CAD build for the part. Positions are in the model's coordinates, mm. Face numbers are marked on the shaded views. A direction names the side the tool comes from. Coordinates: 2 decimals unless noted, no trailing zeros. Loops run counter-clockwise (first coordinate to the right, second up) from the corner with the lowest first, then second, coordinate; pieces in that order, holes last. Notation, with made-up numbers: (55.5, 13.5) -> (92.5, 13.5) arc R36 ccw to (92.5, 49.5) -> close; hole circle Ø7 at (-11.5, 29.25). An arc over 180 degrees is marked (long way). Return JSON: item names as keys, results as strings. Group by question number.
(1) Probe L1, parallel to Z at x = -4.5, y = -6; L2, parallel to Y at x = -8.5, z = 17.1; L3, parallel to X at y = 2, z = 4. List the from-to ranges inside material, lowest first.
(2) Flat gauge pins, fed straight in: pin 1 Ø2 at (y, z) = (15.5, 18) entering from +X; pin 2 Ø4 at (x, z) = (0, 10) entering from +Y; pin 3 Ø1.5 at (y, z) = (-8, 8.5) entering from +X. Where does each tip first touch, or does it go through?
(3) Saw through at B-B on z = 16.5. Write the cut outline in (x, y), then the cut area to 3 significant figures.
(4) Saw through at D-D on x = 0. Write the cut outline in (y, z), then the cut area to 3 significant figures.
(5) Mould opens along Y. For the marked faces 6, 7 and 8 say: pulls with the +Y half, pulls with the -Y half, needs draft (parallel to the pull), parting line crosses it, or undercut.
(6) Saw through at C-C on y = -3. Write the cut outline in (x, z).
(7) Saw through at A-A on x = -8.5. Write the cut outline in (y, z).
(8) Tool access for the marked faces 1, 2, 3, 4 and 5: list every direction of +Z, -Z, +X, -X, +Y, -Y with a clear straight run to the whole face (end or side of a thin tool).
```python
from build123d import *

# Parameters (mm, degrees)
SKETCH_W     = 17
SKETCH_H     = 14
SKETCH_R     = 2.5
PAD_DEPTH    = 3
SKETCH001_W  = 3
SKETCH001_H  = 14
PAD001_DEPTH = 16
SKETCH002_W  = 14
SKETCH002_H  = 3
PAD002_DEPTH = 13
SKETCH003_W  = 34
SKETCH003_H  = 3
PAD003_DEPTH = 9
SKETCH004_W  = 14
SKETCH004_H  = 3
PAD004_DEPTH = 8
SKETCH006_R  = 2
POCKET_DEPTH = 19.001
PAD005_DEPTH = 3
SKETCH008_W  = 23
SKETCH008_H  = 19
PAD006_DEPTH = 3
SKETCH009_W  = 3
SKETCH009_H  = 19
PAD007_DEPTH = 4
CHAMFER_SIZE = 2.9
FILLET_R     = 2
FILLET001_R  = 2
FILLET002_R  = 0.5


with BuildPart() as part:
    # Sketch → Pad (new body)
    with BuildSketch(Plane.XY):
        with Locations((3.5, 0)):
            Rectangle(SKETCH_W, SKETCH_H)
        Circle(SKETCH_R, mode=Mode.SUBTRACT)
    extrude(amount=PAD_DEPTH)

    # Sketch001 (on Face7 of Pad) → Pad001 (join)
    with BuildSketch(Plane.XY.offset(3)):
        with Locations((10.5, 0)):
            Rectangle(SKETCH001_W, SKETCH001_H)
    extrude(amount=PAD001_DEPTH)

    # Sketch002 (on Face10 of Pad001) → Pad002 (join)
    with BuildSketch(Plane(origin=(9, 0, 0), x_dir=(0, -1, 0), z_dir=(-1, 0, 0))):
        with Locations((0, 17.5)):
            Rectangle(SKETCH002_W, SKETCH002_H)
    extrude(amount=PAD002_DEPTH)

    # Sketch003 (on Face16 of Pad002) → Pad003 (join)
    with BuildSketch(Plane(origin=(-4, 0, 0), x_dir=(0, -1, 0), z_dir=(-1, 0, 0))):
        with Locations((-10, 17.5)):
            Rectangle(SKETCH003_W, SKETCH003_H)
    extrude(amount=PAD003_DEPTH)

    # Sketch004 (on Face2 of Pad003) → Pad004 (join)
    with BuildSketch(Plane(origin=(-5, 0, 0), x_dir=(0, -1, 0), z_dir=(-1, 0, 0))):
        with Locations((0, 1.5)):
            Rectangle(SKETCH004_W, SKETCH004_H)
    extrude(amount=PAD004_DEPTH)

    # Sketch006 → Pocket (cut, through all)
    with BuildSketch(Plane.XY.offset(19)):
        with Locations((-8.5, 22)):
            Circle(SKETCH006_R)
        with Locations((-8.5, 12)):
            Circle(SKETCH006_R)
    extrude(amount=-POCKET_DEPTH, mode=Mode.SUBTRACT)

    # Sketch007 (on Face26 of Pocket) → Pad005 (join)
    with BuildSketch(Plane(origin=(-13, 0, 0), x_dir=(0, -1, 0), z_dir=(-1, 0, 0))):
        Polygon((-27, 19), (7, 19), (7, 0), (-7, 0), (-27, 16), align=None)
    extrude(amount=PAD005_DEPTH)

    # Sketch008 (on Face10 of Pad005) → Pad006 (join)
    with BuildSketch(Plane.XZ.offset(7)):
        with Locations((-4.5, 9.5)):
            Rectangle(SKETCH008_W, SKETCH008_H)
    extrude(amount=PAD006_DEPTH)

    # Sketch009 (on Face15 of Pad006) → Pad007 (join)
    with BuildSketch(Plane(origin=(9, 0, 0), x_dir=(0, -1, 0), z_dir=(-1, 0, 0))):
        with Locations((5.5, 9.5)):
            Rectangle(SKETCH009_W, SKETCH009_H)
    extrude(amount=PAD007_DEPTH)

    # Chamfer
    chamfer_edges = [part.edges().sort_by_distance(p)[0] for p in [
        (5, -4, 9.5),
    ]]
    chamfer(chamfer_edges, length=CHAMFER_SIZE)

    # Fillet
    fillet_edges = [part.edges().sort_by_distance(p)[0] for p in [
        (-4, 27, 17.5),
    ]]
    fillet(fillet_edges, radius=FILLET_R)

    # Fillet001
    fillet001_edges = [part.edges().sort_by_distance(p)[0] for p in [
        (-16, 27, 17.5),
    ]]
    fillet(fillet001_edges, radius=FILLET001_R)

    # Fillet002
    fillet002_edges = [part.edges().sort_by_distance(p)[0] for p in [
        (-16, 9, 19),
    ]]
    fillet(fillet002_edges, radius=FILLET002_R)


solid = part.part
```
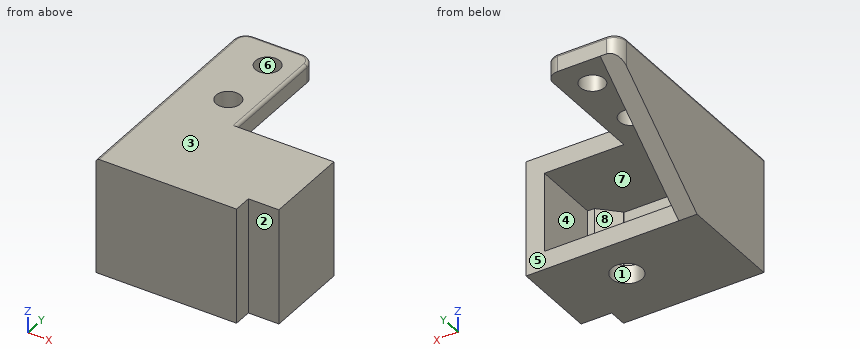
Geometry results:
{
 "1": {"L1": "0 to 3, 16 to 19", "L2": "-10 to 10, 14 to 20, 24 to 27", "L3": "-16 to -13, 9 to 12"},
 "2": {"pin 1": "x = -4", "pin 2": "y = -7", "pin 3": "x = 7"},
 "3": {"outline": "(-16, -10) -> (7, -10) -> (7, -7) -> (12, -7) -> (12, 7) -> (-4, 7) -> (-4, 25) arc R2 ccw to (-6, 27) -> (-14, 27) arc R2 ccw to (-16, 25) -> close; hole circle Ø4 at (-8.5, 12); hole circle Ø4 at (-8.5, 22)", "area": "674 mm²"},
 "4": {"outline": "(-10, 0) -> (-2.5, 0) -> (-2.5, 3) -> (-7, 3) -> (-7, 16) -> (7, 16) -> (7, 19) -> (-10, 19) -> close; (2.5, 0) -> (7, 0) -> (7, 3) -> (2.5, 3) -> close", "area": "126 mm²"},
 "5": {"face 6": "undercut", "face 7": "needs draft", "face 8": "pulls with the +Y half"},
 "6": {"outline": "(-16, 0) -> (12, 0) -> (12, 19) -> (-15.5, 19) arc R0.5 ccw to (-16, 18.5) -> close; hole (-13, 3) -> (9, 3) -> (9, 16) -> (-13, 16) -> close"},
 "7": {"outline": "(-10, 0) -> (7, 0) -> (7, 3) -> (-7, 3) -> (-7, 16) -> (10, 16) -> (10, 19) -> (-10, 19) -> close; (14, 16) -> (20, 16) -> (20, 19) -> (14, 19) -> close; (24, 16) -> (27, 16) -> (27, 18.5) arc R0.5 ccw to (26.5, 19) -> (24, 19) -> close"},
 "8": {"face 1": "-Z", "face 2": "+Z, -Z, +X, -Y", "face 3": "+Z, +X, -X, +Y, -Y", "face 4": "+Y", "face 5": "-Z, +X, +Y"}
}
